from build123d import *

# Parameters (mm, degrees)
F0_R     = 4
F1_DEPTH = 9
F2_R     = 5


with BuildPart() as f1:
    # F0 (on Top) → F1 (new body)
    with BuildSketch(Plane.XY):
        with BuildLine():
            Line((-40.391175, 44.074847), (-8, 30))
            Line((-8, 30), (-8, 45))
            Line((-8, 45), (21, 45))
            Line((21, 45), (-36.931732, 55.481916))
            ThreePointArc((-36.931732, 55.481916), (-33.395132, 53.424234), (-32, 49.577781))
            ThreePointArc((-32, 49.577781), (-34.709639, 44.560459), (-40.391175, 44.074847))
        make_face()
        with BuildLine():
            ThreePointArc((-36.931732, 55.481916), (-43.741761, 51.319096), (-40.391175, 44.074847))
            ThreePointArc((-40.391175, 44.074847), (-34.709639, 44.560459), (-32, 49.577781))
            ThreePointArc((-32, 49.577781), (-33.395132, 53.424234), (-36.931732, 55.481916))
        make_face()
        with Locations((-38, 49.577781)):
            Circle(F0_R, mode=Mode.SUBTRACT)
        Polygon((-8, 0), (0, 0), (0, 35), (13, 35), (13, 0), (21, 0), (21, 45), (-8, 45), (-8, 30), align=None)
    extrude(amount=F1_DEPTH)

    # F2
    f2_edges = [f1.edges().sort_by_distance(p)[0] for p in [
        (-8, 30, 4.5),
        (21, 45, 4.5),
        (-8, 0, 4.5),
        (21, 0, 4.5),
    ]]
    fillet(f2_edges, radius=F2_R)


solid = f1.part
Check sheet for the modelled part. Datum: model origin and axes. Units: mm. A direction names the side the tool comes from. Round coordinates to 2 decimals unless told otherwise and drop trailing zeros. Loops run counter-clockwise (first coordinate to the right, second up) from the corner with the lowest first, then second, coordinate; pieces in that order, holes last.
1. Gauge pin test, flat ends, axial feed: pin 1 Ø2 at (x, z) = (7, 2) entering from -Y; pin 2 Ø2.5 at (y, z) = (15.5, 6.5) entering from -X; pin 3 Ø3 at (x, z) = (-29.5, 5.5) entering from +Y. Record the tip position at first contact, or that the pin passes through.
2. Sectioned sample at C-C on x = -38. Record the boundary of the cut face in (y, z), and give its area (3 significant figures).
3. Set-up check for faces 1 (the flat face through (21, 23, 4)), 2 (the flat face through (-8, 16, 4)), 3 (the flat face through (0, 17, 4)): record each of +Z, -Z, +X, -X, +Y, -Y from which the full face is reachable in a straight line by a thin tool's end or side.
4. Sectioned sample at A-A on y = 10. Record the boundary of the cut face in (x, z).
5. Sectioned sample at D-D on y = 43. Record the boundary of the cut face in (x, z).
6. Mould release check, pull along X, two halves, no side actions. Record for faces 4 (the flat face through (-5, 34, 9)), 5 (the cylindrical face through (-38.867, 45.673, 4.437)), 6 (the cylindrical face through (19, 1, 5)): released by +X, released by -X, zero draft, split by the parting line, or undercut.
7. Sectioned sample at B-B on z = 7.25. Record the boundary of the cut face in (x, y), and give its area (3 significant figures).
8. Scan lines: probe 1 along X at (y, z) = (18, 7.5); probe 2 along Y at (x, z) = (-38, 6.75); probe 3 along X at (y, z) = (28, 7). Record each from-to range of solid material in increasing order.
Recorded:
1. pin 1: stops at y = 35
1. pin 2: stops at x = -8
1. pin 3: stops at y = 54.41
2. outline: (43.04, 0) - (45.58, 0) - (45.58, 9) - (43.04, 9) - close; (53.58, 0) - (55.58, 0) - (55.58, 9) - (53.58, 9) - close
2. area: 40.9 mm2
3. face 1: +Z, -Z, +X, +Y, -Y
3. face 2: +Z, -Z, -X, -Y
3. face 3: +Z, -Z, -Y
4. outline: (-8, 0) - (0, 0) - (0, 9) - (-8, 9) - close; (13, 0) - (21, 0) - (21, 9) - (13, 9) - close
5. outline: (-37.92, 0) - (20.5, 0) - (20.5, 9) - (-37.92, 9) - close
6. face 4: zero draft
6. face 5: undercut
6. face 6: released by +X
7. outline: (-40.39, 44.07) - (-11.01, 31.31) arc R5 cw to (-8, 26.72) - (-8, 5) arc R5 ccw to (-3, 0) - (0, 0) - (0, 35) - (13, 35) - (13, 0) - (16, 0) arc R5 ccw to (21, 5) - (21, 40.82) arc R5 ccw to (16.89, 45.74) - (-36.93, 55.48) arc R6 ccw to start; hole circle Ø8 at (-38, 49.58)
7. area: 1,410 mm2
8. probe 1: x = -8 to 0, 13 to 21
8. probe 2: y = 43.04 to 45.58, 53.58 to 55.58
8. probe 3: x = -8.17 to 0, 13 to 21
